Geometry check sheet. Reference: the model listing, model coordinates, mm. Coordinates: 2 decimals unless noted, no trailing zeros. Write each loop counter-clockwise with the first axis right and the second up, starting at its lowest first coordinate (ties: lowest second). Pieces come first, ordered by that corner, then holes. Notation, with made-up numbers: (-13, 13) -> (6, 13) arc R10 cw to (6, 30) -> close; hole circle Ø4 at (89, -36). An arc over 180 degrees is marked (long way). Answer in a Markdown table with one row per item. Add a question column.
1. Cross-section at C-C on z = 3. Record the cut outline in (x, y).
2. Cross-section at A-A on y = 0. Record the cut outline in (x, z).
3. Scan lines: L1, parallel to Y at x = -15, z = 2.5; L2, parallel to X at y = -17, z = 1.95; L3, parallel to Y at x = 0, z = 1.95. Record each from-to range of solid material in increasing order. Write a range as from..to.
4. Cross-section at D-D on y = -21.5. Record the cut outline in (x, z), and give its area (3 significant figures).
5. Mould release check, pull along X, two halves, no side actions. Record for faces 1 (the flat face through (6, -6, 4)), 2 (the cylindrical face through (-5.961, -26.846, 1.972)), 3 (the cylindrical face through (17.8, -16.74, 2.03)): pulls with the +X half, pulls with the -X half, needs draft (parallel to the pull), parting line crosses it, or undercut.
6. Depth check by flat-ended pin: P1, Ø3.5, axis at x = -16.05, y = 16.02, coming from the -Z side; P2, Ø1, axis at y = -16, z = 1, coming from the -X side; P3, Ø1.5, axis at x = -13.5, z = 1, coming from the -Y side. Enter the tip coordinate at first touch or a pass-through.
```python
from build123d import *

# Parameters (mm, degrees)
SKETCH1_R           = 27.5
BOSS_EXTRUDE1_DEPTH = 4
CUT_EXTRUDE1_DEPTH  = 4
SKETCH3_R           = 7
CUT_EXTRUDE2_DEPTH  = 4


with BuildPart() as part:
    # Sketch1 → Boss-Extrude1 (new body)
    with BuildSketch(Plane.XY):
        Circle(SKETCH1_R)
    extrude(amount=BOSS_EXTRUDE1_DEPTH)

    # Sketch2 → Cut-Extrude1 (cut)
    with BuildSketch(Plane.XY.offset(4)):
        with BuildLine():
            ThreePointArc((-14.049415004, 16.024707502), (-16.049415004, 18.024707502), (-18.049415004, 16.024707502))
            ThreePointArc((-18.049415004, 16.024707502), (-16.049415004, 14.024707502), (-14.049415004, 16.024707502))
        make_face()
        with BuildLine():
            ThreePointArc((-14.049415004, -15.975292498), (-16.049415004, -13.975292498), (-18.049415004, -15.975292498))
            ThreePointArc((-18.049415004, -15.975292498), (-16.049415004, -17.975292498), (-14.049415004, -15.975292498))
        make_face()
        with BuildLine():
            ThreePointArc((13.950584996, -15.975292498), (15.950584996, -17.975292498), (17.950584996, -15.975292498))
            ThreePointArc((17.950584996, -15.975292498), (15.950584996, -13.975292498), (13.950584996, -15.975292498))
        make_face()
        with BuildLine():
            ThreePointArc((13.950584996, 16.024707502), (15.950584996, 14.024707502), (17.950584996, 16.024707502))
            ThreePointArc((17.950584996, 16.024707502), (15.950584996, 18.024707502), (13.950584996, 16.024707502))
        make_face()
    extrude(amount=-CUT_EXTRUDE1_DEPTH, mode=Mode.SUBTRACT)

    # Sketch3 → Cut-Extrude2 (cut)
    with BuildSketch(Plane.XY.offset(4)):
        Circle(SKETCH3_R)
    extrude(amount=-CUT_EXTRUDE2_DEPTH, mode=Mode.SUBTRACT)


solid = part.part
```
Results found:
| question | item | result |
|---|---|---|
| 1 | outline | circle Ø55 at (0, 0); hole circle Ø4 at (-16.05, -15.98); hole circle Ø4 at (-16.05, 16.02); hole circle Ø14 at (0, 0); hole circle Ø4 at (15.95, -15.98); hole circle Ø4 at (15.95, 16.02) |
| 2 | outline | (-27.5, 0) -> (-7, 0) -> (-7, 4) -> (-27.5, 4) -> close; (7, 0) -> (27.5, 0) -> (27.5, 4) -> (7, 4) -> close |
| 3 | L1 | y = -23.05..-17.68, -14.27..14.32, 17.73..23.05 |
| 3 | L2 | x = -21.62..-17.77, -14.33..14.23, 17.67..21.62 |
| 3 | L3 | y = -27.5..-7, 7..27.5 |
| 4 | outline | (-17.15, 0) -> (17.15, 0) -> (17.15, 4) -> (-17.15, 4) -> close |
| 4 | area | 137 mm^2 |
| 5 | face 1 | needs draft |
| 5 | face 2 | parting line crosses it |
| 5 | face 3 | undercut |
| 6 | P1 | passes through |
| 6 | P2 | stops at x = -22.72 |
| 6 | P3 | stops at y = -24.37 |
